Work out the finished part from the listing and answer in its coordinate system (mm). A direction names the side the tool comes from. Round coordinates to 2 decimals unless told otherwise and drop trailing zeros. Order: outer loops, then holes, each group sorted by start corner. A loop starts at its lowest first (then second) coordinate and runs counter-clockwise, first axis right, second up. Notation, with made-up numbers: (-1, -38) -> (25, -38) arc R32 ccw to (25, -1) -> close; hole circle Ø7 at (-25.75, -16.5). An arc over 180 degrees is marked (long way). Use one line per item in the form item = value.
```python
from build123d import *

# Parameters (mm, degrees)
SKETCH001_R     = 5
PAD001_DEPTH    = 35
SKETCH_W        = 70
SKETCH_H        = 67.4
PAD_DEPTH       = 5
SKETCH002_W     = 10
SKETCH002_H     = 5
POCKET_DEPTH    = 10.001
SKETCH003_R     = 6.85
POCKET001_DEPTH = 21.7


with BuildPart() as pad001:
    # Sketch001 → Pad001 (new body, symmetric)
    with BuildSketch(Plane.XZ):
        with Locations((-38.5, 0)):
            Circle(SKETCH001_R)
        with Locations((38.5, 0)):
            Circle(SKETCH001_R)
    extrude(amount=PAD001_DEPTH, both=True)


with BuildPart() as pocket001:
    # Sketch → Pad (new body, symmetric)
    with BuildSketch(Plane.XY):
        Rectangle(SKETCH_W, SKETCH_H)
    extrude(amount=PAD_DEPTH, both=True)

    # Cut: cut Pad001
    add(pad001.part, mode=Mode.SUBTRACT)

    # Sketch002 → Pocket (cut, through all)
    with BuildSketch(Plane.XY.offset(5)):
        with Locations((0, 27.5)):
            Rectangle(SKETCH002_W, SKETCH002_H)
    extrude(amount=-POCKET_DEPTH, mode=Mode.SUBTRACT)

    # Sketch003 → Pocket001 (cut)
    with BuildSketch(Plane(origin=(0, 33.7, 0), x_dir=(-1, 0, 0), z_dir=(0, 1, 0))):
        with Locations((-39.7, 0)):
            Circle(SKETCH003_R)
        with Locations((39.7, 0)):
            Circle(SKETCH003_R)
    extrude(amount=-POCKET001_DEPTH, mode=Mode.SUBTRACT)


solid = pocket001.part
```
Item 1: Determine the mould class of faces 5 (the flat face through (0, 0, -5)), 6 (the cylindrical face through (33.5, -11.2, 0.1)), 7 (the flat face through (0, 0, 5)) for opening direction Z: released by +Z, released by -Z, zero draft, split by the parting line, or undercut.
Findings:
face_5 = released by -Z
face_6 = undercut
face_7 = released by +Z
Item 2: For faces 1 (the flat face through (5, 27, 0)), 2 (the cylindrical face through (-32.85, 23, 0.08)), 3 (the flat face through (0, 33.7, 0)), 4 (the cylindrical face through (32.85, 23, -0.08)), determine the directions among +Z, -Z, +X, -X, +Y, -Y from which every point of the face is accessible in a straight line to the end or side of a thin tool.
Findings:
face_1 = +Z, -Z
face_2 = -X, +Y
face_3 = +Z, -Z, +X, -X, +Y
face_4 = +X, +Y
Item 3: Consider line 1 along Y through (x, z) = (-4, -2); line 2 along X through (y, z) = (-8, -1.25); line 3 along X through (y, z) = (-9, 2). Determine where each line is inside the solid, lowest interval first.
Findings:
line_1 = -33.7 to 25, 30 to 33.7
line_2 = -33.66 to 33.66
line_3 = -33.92 to 33.92
Item 4: The part is cut by section C-C, the plane y = -2.5. Give the vertices of the cut face in (x, z).
Findings:
outline = (-35, -5) -> (35, -5) -> (35, -3.57) arc R5 cw to (35, 3.57) -> (35, 5) -> (-35, 5) -> (-35, 3.57) arc R5 cw to (-35, -3.57) -> close
Item 5: The part is cut by section B-B, the plane z = 0.25. Give the vertices of the cut face in (x, y).
Findings:
outline = (-33.51, -33.7) -> (33.51, -33.7) -> (33.51, 12) -> (32.85, 12) -> (32.85, 33.7) -> (-32.85, 33.7) -> (-32.85, 12) -> (-33.51, 12) -> close; hole (-5, 25) -> (5, 25) -> (5, 30) -> (-5, 30) -> close
Item 6: Flat-ended cylindrical pins translate along their axes: P1, Ø3, axis at y = 10, z = -2, coming from the -X side; P2, Ø4, axis at y = -18.5, z = 1.5, coming from the +X side; P3, Ø1.5, axis at y = 27, z = 2, coming from the -X side. Find the tip coordinate at first contact, or state that the pin passes through.
Findings:
P1 = -34.93
P2 = 34.93
P3 = -33.43
